from build123d import *

# Parameters (mm, degrees)
BOX004_W                    = 5
BOX004_H                    = 5
BOX004_DEPTH                = 5
CYLINDER001_W               = 48
CYLINDER001_H               = 15
CYLINDER001_ANGLE           = 60
CYLINDER001_PLACEMENT_ANGLE = 60
CYLINDER_W                  = 52
CYLINDER_H                  = 15
CYLINDER_ANGLE              = 60
CYLINDER_PLACEMENT_ANGLE    = 60
BOX003_W                    = 6
BOX003_H                    = 4
BOX003_DEPTH                = 15
BOX002_W                    = 10
BOX002_H                    = 10
BOX002_DEPTH                = 15
BOX001_W                    = 13
BOX001_H                    = 27
BOX001_DEPTH                = 12
BOX_W                       = 16
BOX_H                       = 40
BOX_DEPTH                   = 14


with BuildPart() as pin_opening:
    # Box004 → Box004 (new body)
    with BuildSketch(Plane(origin=(6, 38.5, 5), x_dir=(1, 0, 0), z_dir=(0, 0, 1))):
        with Locations((2.5, 2.5)):
            Rectangle(BOX004_W, BOX004_H)
    extrude(amount=BOX004_DEPTH)


with BuildPart() as bottle_wall001:
    # Cylinder001 → Cylinder001 (revolve)
    with BuildSketch(Plane.XZ):
        with Locations((24, 7.5)):
            Rectangle(CYLINDER001_W, CYLINDER001_H)
    revolve(axis=Axis((0, 0, 0), (0, 0, 1)), revolution_arc=CYLINDER001_ANGLE)


with BuildPart() as bottle_wall001_1:
    # Cylinder001 placement: moved
    add(bottle_wall001.part.moved(Location((8.5, -7, 0))).rotate(Axis((8.5, -7, 0), (0, 0, 1)), CYLINDER001_PLACEMENT_ANGLE))


with BuildPart() as cut005:
    # Cylinder → Cylinder (revolve)
    with BuildSketch(Plane.XZ):
        with Locations((26, 7.5)):
            Rectangle(CYLINDER_W, CYLINDER_H)
    revolve(axis=Axis((0, 0, 0), (0, 0, 1)), revolution_arc=CYLINDER_ANGLE)


with BuildPart() as cut005_1:
    # Cylinder placement: moved
    add(cut005.part.moved(Location((8.5, -7, 0))).rotate(Axis((8.5, -7, 0), (0, 0, 1)), CYLINDER_PLACEMENT_ANGLE))

    # Cut005: cut bottle_wall001
    add(bottle_wall001_1.part, mode=Mode.SUBTRACT)


with BuildPart() as cut005_2:
    # Cut005 placement: moved
    add(cut005_1.part.moved(Location((0, -2, 0))))


with BuildPart() as cone:
    # Cone → Cone (revolve)
    with BuildSketch(Plane(origin=(8.5, 1, 2), x_dir=(1, 0, 0), z_dir=(0, -1, 0))):
        Polygon((0, 0), (1, 0), (2, 5), (0, 5), align=None)
    revolve(axis=Axis((8.5, 1, 2), (0, 0, 1)))


with BuildPart() as pinhole:
    # Sphere → Sphere (revolve)
    with BuildSketch(Plane(origin=(8.5, 1.25, 7), x_dir=(1, 0, 0), z_dir=(0, -1, 0))):
        with BuildLine():
            ThreePointArc((0, -2.5), (2.5, 0), (0, 2.5))
            Line((0, 2.5), (0, -2.5))
        make_face()
    revolve(axis=Axis((8.5, 1.25, 7), (0, 0, 1)))


with BuildPart() as neck:
    # Box003 → Box003 (new body)
    with BuildSketch(Plane(origin=(5.5, 28, 4), x_dir=(1, 0, 0), z_dir=(0, 0, 1))):
        with Locations((3, 2)):
            Rectangle(BOX003_W, BOX003_H)
    extrude(amount=BOX003_DEPTH)


with BuildPart() as pullbay:
    # Box002 → Box002 (new body)
    with BuildSketch(Plane(origin=(3.5, 30, 2), x_dir=(1, 0, 0), z_dir=(0, 0, 1))):
        with Locations((5, 5)):
            Rectangle(BOX002_W, BOX002_H)
    extrude(amount=BOX002_DEPTH)


with BuildPart() as solenoidbay:
    # Box001 → Box001 (new body)
    with BuildSketch(Plane(origin=(2, 2, 2), x_dir=(1, 0, 0), z_dir=(0, 0, 1))):
        with Locations((6.5, 13.5)):
            Rectangle(BOX001_W, BOX001_H)
    extrude(amount=BOX001_DEPTH)


with BuildPart() as cut006:
    # Box → Box (new body)
    with BuildSketch(Plane.XY):
        with Locations((8, 20)):
            Rectangle(BOX_W, BOX_H)
    extrude(amount=BOX_DEPTH)

    # Cut: cut solenoidBay
    add(solenoidbay.part, mode=Mode.SUBTRACT)

    # Cut001: cut pullBay
    add(pullbay.part, mode=Mode.SUBTRACT)

    # Cut002: cut neck
    add(neck.part, mode=Mode.SUBTRACT)

    # Cut003: cut pinhole
    add(pinhole.part, mode=Mode.SUBTRACT)

    # Cut004: cut Cone
    add(cone.part, mode=Mode.SUBTRACT)

    # Fusion: union Cut005
    add(cut005_2.part)

    # Cut006: cut pin_opening
    add(pin_opening.part, mode=Mode.SUBTRACT)


solid = cut006.part
Input: part model. Units: mm. Frame: model coordinates. A direction names the side the tool comes from. Coordinates: 2 decimals unless noted, no trailing zeros. Loops run counter-clockwise (first coordinate to the right, second up) from the corner with the lowest first, then second, coordinate; pieces in that order, holes last.
Q1. Cut plane A-A (z = 6.25). Output: boundary loops of the cut face in (x, y).
Q2. Cut plane B-B (y = 26). Output: boundary loops of the cut face in (x, z).
Q3. Cut plane D-D (x = 12.5). Output: boundary loops of the cut face in (y, z).
Q4. Material intervals for line 1 (Y direction, x = 9.5, z = 11); line 2 (X direction, y = 6, z = 4.25); line 3 (Z direction, x = 14.5, y = 22), sorted ascending.
Q5. Cut plane C-C (z = 13). Output: boundary loops of the cut face in (x, y), then the cut area to 3 significant figures.
Q6. Contact query for flat-ended pins moving along their axis: pin 1 (2 mm diameter, centred on y = 21.5, z = 13, fed in from -X); pin 2 (1.6 mm diameter, centred on x = 8, y = 0.5, fed in from +Z); pin 3 (5 mm diameter, centred on x = 10, y = 19, fed in from +Z). Output: stop coordinate, or through.
Q7. Draft query along Y for faces 4 (the face through (8, 24, 0)), 5 (the face through (33.5, 34.3, 7.6)), 6 (the face through (8, 16, 2)). Return one class per face: +Y half, -Y half, draft (parallel to the pull), parting line (faces both ways), or undercut.
Q8. Set-up query: faces 1 (the face through (6, 41, 7)), 2 (the face through (9.9, 2, 9.2)), 3 (the face through (9.76, 0.97, 3.3)). Return all of +Z, -Z, +X, -X, +Y, -Y with unobstructed straight access to the full face (end or side cutting, diameter ignored); none if empty.
Working result:
1. outline: (-17.5, 36.03) - (-15.5, 32.57) arc R48 cw to (0, 38.24) - (0, 0) - (6.47, 0) arc R2.38 cw to (6.24, 2) - (2, 2) - (2, 29) - (5.5, 29) - (5.5, 30) - (3.5, 30) - (3.5, 38.74) arc R48 cw to (6, 38.93) - (6, 42.94) arc R52 ccw to start; (10.53, 0) - (16, 0) - (16, 38.41) arc R48 cw to (32.5, 32.57) - (34.5, 36.03) arc R52 ccw to (11, 42.94) - (11, 38.93) arc R48 cw to (13.5, 38.74) - (13.5, 30) - (11.5, 30) - (11.5, 29) - (15, 29) - (15, 2) - (10.76, 2) arc R2.38 cw to start
2. outline: (0, 0) - (16, 0) - (16, 14) - (15, 14) - (15, 2) - (2, 2) - (2, 14) - (0, 14) - close
3. outline: (0, 0) - (42.85, 0) - (42.85, 15) - (38.83, 15) - (38.83, 2) - (30, 2) - (30, 14) - (29, 14) - (29, 2) - (2, 2) - (2, 14) - (0, 14) - close
4. line 1: y = 0 to 2, 38.99 to 42.99
4. line 2: x = 0 to 2, 15 to 16
4. line 3: z = 0 to 2
5. outline: (-17.5, 36.03) - (-15.5, 32.57) arc R48 cw to (0, 38.24) - (0, 0) - (16, 0) - (16, 38.41) arc R48 cw to (32.5, 32.57) - (34.5, 36.03) arc R52 ccw to start; hole (2, 2) - (15, 2) - (15, 29) - (11.5, 29) - (11.5, 30) - (13.5, 30) - (13.5, 38.74) arc R48 ccw to (3.5, 38.74) - (3.5, 30) - (5.5, 30) - (5.5, 29) - (2, 29) - close
5. area: 384 mm2
6. pin 1: stops at x = 0
6. pin 2: stops at z = 14
6. pin 3: stops at z = 2
7. face 4: draft
7. face 5: -Y half
7. face 6: undercut
8. face 1: +Y
8. face 2: +Z
8. face 3: none
